The model under review builds one solid part; all positions refer to its coordinate system, in mm. Coordinates: 2 decimals unless noted, no trailing zeros. Order: outer loops, then holes, each group sorted by start corner. A loop starts at its lowest first (then second) coordinate and runs counter-clockwise, first axis right, second up. Notation, with made-up numbers: M 51.5,40.25 L 63.5,40.25 A24 ccw 63.5,65.25 Z; hole C 16,48 d6. An arc over 180 degrees is marked long. Answer as CSV lines item,"result". Start each with the question number.
Q1. Consider section B-B on y = 0. Write out the cut boundary in (x, z).
Q2. For P1, Ø12, axis at x = -10.5, z = 8, coming from the +Y side; P2, Ø5.5, axis at y = 0, z = 45, coming from the -X side; P3, Ø1.5, axis at y = -8.5, z = 7.5, coming from the -X side; P4, Ø1, axis at y = -12, z = 7.5, coming from the +X side, all flat-tipped, find the tip position at first contact; note any pin that passes through.
Q3. Consider section C-C on x = 0. Write out the cut boundary in (y, z), and give its area (3 significant figures).
Q4. Consider section D-D on y = 15. Write out the cut boundary in (x, z), and give its area (3 significant figures).
Q5. Wall thickness on L1, parallel to X at y = 8, z = 42.5; L2, parallel to X at y = -14, z = 31.5; L3, parallel to Y at x = 7, z = 2.5: over which ranges is each line inside the solid? List them lowest first. Write a range as [from, to].
Q6. The part is to be moulded in two halves that separate along Y. For faces 1 (the face through (-0.1, 25.6, 5)), 2 (the face through (-25.5, -2.1, 12.8)), say which applies: +Y half, -Y half, draft (parallel to the pull), parting line (faces both ways), or undercut.
Q7. Consider section A-A on z = 28.5. Write out the cut boundary in (x, y), and give its area (3 significant figures).
from build123d import *
from build123d.topology import SkipClean

# Parameters (mm, degrees)
SKETCH2_R               = 26
SKETCH2_R_2             = 25.25
BOSS_EXTRUDE1_DEPTH     = 5
BOSS_EXTRUDE2_DEPTH     = 50
CUT_EXTRUDE1_DEPTH      = 67.158899628
CUT_EXTRUDE1_DEPTH_BACK = 67.158899628
SKETCH4_R               = 3.5


with BuildPart() as part:
    # Sketch2 → Boss-Extrude1 (new body)
    with BuildSketch(Plane.XY):
        Circle(SKETCH2_R)
        Circle(SKETCH2_R_2, mode=Mode.SUBTRACT)
    extrude(amount=BOSS_EXTRUDE1_DEPTH)

    # Sketch3 → Boss-Extrude2 (add)
    with SkipClean():  # the faces are left unmerged after this step: merging them gives an invalid solid
        with BuildSketch(Plane.XY.offset(5)):
            with BuildLine():
                Line((-17.854446225, 17.854446225), (-18.384776311, 18.384776311))
                ThreePointArc((-18.384776311, 18.384776311), (-26, 0), (-18.384776311, -18.384776311))
                Line((-18.384776311, -18.384776311), (-17.854446225, -17.854446225))
                ThreePointArc((-17.854446225, -17.854446225), (-25.25, 0), (-17.854446225, 17.854446225))
            make_face()
            with BuildLine():
                Line((17.854446225, -17.854446225), (18.384776311, -18.384776311))
                ThreePointArc((18.384776311, -18.384776311), (26, 0), (18.384776311, 18.384776311))
                Line((18.384776311, 18.384776311), (17.854446225, 17.854446225))
                ThreePointArc((17.854446225, 17.854446225), (25.25, 0), (17.854446225, -17.854446225))
            make_face()
        extrude(amount=BOSS_EXTRUDE2_DEPTH)

    # Sketch4 → Cut-Extrude1 (cut, two sides: drawn at the far end of the back side and taken through both)
    with SkipClean():  # the faces are left unmerged after this step: merging them gives an invalid solid
        with BuildSketch(Plane(origin=(0, 0, 0), x_dir=(0, 0, -1), z_dir=(1, 0, 0)).offset(-CUT_EXTRUDE1_DEPTH_BACK)):
            with Locations((-45, 0)):
                Circle(SKETCH4_R)
            with Locations((-10, 0)):
                Circle(SKETCH4_R)
        extrude(amount=CUT_EXTRUDE1_DEPTH + CUT_EXTRUDE1_DEPTH_BACK, mode=Mode.SUBTRACT)


solid = part.part
Evaluation:
1,outline,"M -26,0 L -25.25,0 L -25.25,6.5 L -26,6.5 Z; M -26,13.5 L -25.25,13.5 L -25.25,41.5 L -26,41.5 Z; M -26,48.5 L -25.25,48.5 L -25.25,55 L -26,55 Z; M 25.25,0 L 26,0 L 26,6.5 L 25.25,6.5 Z; M 25.25,13.5 L 26,13.5 L 26,41.5 L 25.25,41.5 Z; M 25.25,48.5 L 26,48.5 L 26,55 L 25.25,55 Z"
2,P1,"stops at y = 25.45"
2,P2,"passes through"
2,P3,"stops at x = -24.82"
2,P4,"stops at x = 23.32"
3,outline,"M -26,0 L -25.25,0 L -25.25,5 L -26,5 Z; M 25.25,0 L 26,0 L 26,5 L 25.25,5 Z"
3,area,"7.50 mm²"
4,outline,"M -21.24,0 L -20.31,0 L -20.31,55 L -21.24,55 Z; M 20.31,0 L 21.24,0 L 21.24,55 L 20.31,55 Z"
4,area,"102 mm²"
5,L1,"x = [-24.74, -23.95], [23.95, 24.74]"
5,L2,"x = [-21.91, -21.01], [21.01, 21.91]"
5,L3,"y = [-25.04, -24.26], [24.26, 25.04]"
6,face 1,"draft"
6,face 2,"undercut"
7,outline,"M -18.38,-18.38 L -17.85,-17.85 A25.25 cw -17.85,17.85 L -18.38,18.38 A26 ccw Z; M 17.85,-17.85 L 18.38,-18.38 A26 ccw 18.38,18.38 L 17.85,17.85 A25.25 cw Z"
7,area,"60.4 mm²"
